Read the model definition and answer for the solid it produces. Units are mm, in the model's axes. Face numbers are marked on the shaded views. A direction names the side the tool comes from. Coordinates: 2 decimals unless noted, no trailing zeros. Write each loop counter-clockwise with the first axis right and the second up, starting at its lowest first coordinate (ties: lowest second). Pieces come first, ordered by that corner, then holes. Notation, with made-up numbers: (4, 3.25) - (14, 3.25) arc R16 cw to (14, 25.25) - close; hole circle Ø4 at (-2, 34). An arc over 180 degrees is marked (long way). Use a Markdown table: item, result.
from build123d import *

# Parameters (mm, degrees)
F1_DEPTH  = 230
F3_D      = 48.6
F5_D      = 6.5
F6_D      = 5.5
F7_SIZE   = 10
F9_D      = 13.72
F9_DEPTH  = 5
F11_D     = 19.05
F11_DEPTH = 5
F12_D     = 12.7
F12_DEPTH = 5


with BuildPart() as f1:
    # F0 (on Right) → F1 (new body)
    with BuildSketch(Plane.YZ):
        with BuildLine():
            Line((205, 0), (-205, 0))
            ThreePointArc((-205, 0), (-206.414214, -0.585786), (-207, -2))
            Line((-207, -2), (-207, -238))
            Line((-207, -238), (-247, -238))
            Line((-247, -238), (-247, -240))
            Line((-247, -240), (-207, -240))
            ThreePointArc((-207, -240), (-205.585786, -239.414214), (-205, -238))
            Line((-205, -238), (-205, -2))
            Line((-205, -2), (205, -2))
            Line((205, -2), (205, -238))
            ThreePointArc((205, -238), (205.585786, -239.414214), (207, -240))
            Line((207, -240), (247, -240))
            Line((247, -240), (247, -238))
            Line((247, -238), (207, -238))
            Line((207, -238), (207, -2))
            ThreePointArc((207, -2), (206.414214, -0.585786), (205, 0))
        make_face()
    extrude(amount=F1_DEPTH)

    # F3 (through all)
    with Locations(Plane.XY):
        with Locations((115, -162)):
            Hole(F3_D / 2)

    # F5 (through all)
    with Locations(Plane.XY.offset(-238)):
        with Locations((35, -237), (65, -237), (165, -237), (195, -237)):
            Hole(F5_D / 2)

    # F6 (through all)
    with Locations(Plane.XY.offset(-238)):
        with Locations((35, 237), (65, 237), (165, 237), (195, 237)):
            Hole(F6_D / 2)

    # F7
    f7_edges = [f1.edges().sort_by_distance(p)[0] for p in [
        (0, -247, -239),
        (230, -247, -239),
        (230, 247, -239),
        (0, 247, -239),
    ]]
    chamfer(f7_edges, length=F7_SIZE)

    # F9
    with Locations(Plane.XZ.offset(207)):
        with Locations((17.5, -20), (17.5, -200)):
            Hole(F9_D / 2, depth=F9_DEPTH)

    # F11
    with Locations(Plane(origin=(0, 207, 0), x_dir=(-1, 0, 0), z_dir=(0, 1, 0))):
        with Locations((-115, -20)):
            Hole(F11_D / 2, depth=F11_DEPTH)

    # F12
    with Locations(Plane(origin=(0, 207, 0), x_dir=(-1, 0, 0), z_dir=(0, 1, 0))):
        with Locations((-40, -20)):
            Hole(F12_D / 2, depth=F12_DEPTH)


solid = f1.part
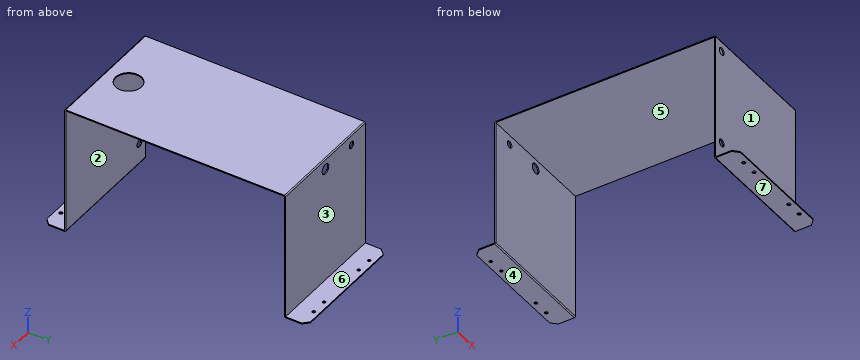
(1) A cutting plane is placed at D-D, the plane x = 182.5. Write down the section's boundary in (y, z), and give its area (3 significant figures).
Report:
| item | result |
|---|---|
| outline | (-247, -240) - (-207, -240) arc R2 ccw to (-205, -238) - (-205, -2) - (205, -2) - (205, -238) arc R2 ccw to (207, -240) - (247, -240) - (247, -238) - (207, -238) - (207, -2) arc R2 ccw to (205, 0) - (-205, 0) arc R2 ccw to (-207, -2) - (-207, -238) - (-247, -238) - close |
| area | 1,940 mm² |
(2) A cutting plane is placed at C-C, the plane z = -150. Write down the section's boundary in (x, y), and give its area (3 significant figures).
Report:
| item | result |
|---|---|
| outline | (0, -207) - (230, -207) - (230, -205) - (0, -205) - close; (0, 205) - (230, 205) - (230, 207) - (0, 207) - close |
| area | 920 mm² |
(3) A cutting plane is placed at A-A, the plane z = -20. Write down the section's boundary in (x, y) (3 decimals).
Report:
| item | result |
|---|---|
| outline | (0, -207) - (10.64, -207) - (10.64, -205) - (0, -205) - close; (0, 205) - (33.65, 205) - (33.65, 207) - (0, 207) - close; (24.36, -207) - (230, -207) - (230, -205) - (24.36, -205) - close; (46.35, 205) - (105.475, 205) - (105.475, 207) - (46.35, 207) - close; (124.525, 205) - (230, 205) - (230, 207) - (124.525, 207) - close |
(4) Straight lines are drawn through the part: L1, parallel to X at y = 237, z = -239.2; L2, parallel to Y at x = 79.5, z = -229; L3, parallel to X at y = -237, z = -238.9. For each, find the intervals that lie inside material, in ascending order.
Report:
| item | result |
|---|---|
| L1 | x = 0 to 32.25, 37.75 to 62.25, 67.75 to 162.25, 167.75 to 192.25, 197.75 to 230 |
| L2 | y = -207 to -205, 205 to 207 |
| L3 | x = 0 to 31.75, 38.25 to 61.75, 68.25 to 161.75, 168.25 to 191.75, 198.25 to 230 |
(5) The mould has two halves that part along Y. Classify the marked faces 1, 2, 3 and 4: pulls with the +Y half, pulls with the -Y half, needs draft (parallel to the pull), parting line crosses it, or undercut.
Report:
| item | result |
|---|---|
| face 1 | pulls with the -Y half |
| face 2 | undercut |
| face 3 | pulls with the +Y half |
| face 4 | needs draft |
(6) Each of these flat-tipped pins is pushed along its axis until it touches: P1, Ø5, axis at x = 165, y = 237, coming from the -Z side; P2, Ø10.5, axis at x = 165, y = -237, coming from the -Z side; P3, Ø10, axis at x = 155.5, z = -215, coming from the -Y side; P4, Ø6, axis at x = 160, z = -126, coming from the +Y side. Where does it stop, or does it pass through?
Report:
| item | result |
|---|---|
| P1 | passes through |
| P2 | stops at z = -240 |
| P3 | stops at y = -207 |
| P4 | stops at y = 207 |
(7) For the marked faces 5, 6 and 7, determine the directions among +Z, -Z, +X, -X, +Y, -Y from which every point of the face is accessible in a straight line to the end or side of a thin tool.
Report:
| item | result |
|---|---|
| face 5 | -Z, +X, -X |
| face 6 | +Z, +X, -X, +Y |
| face 7 | -Z, +X, -X, +Y, -Y |
(8) A cutting plane is placed at B-B, the plane x = 115. Write down the section's boundary in (y, z) (3 decimals).
Report:
| item | result |
|---|---|
| outline | (-247, -240) - (-207, -240) arc R2 ccw to (-205, -238) - (-205, -2) - (-186.3, -2) - (-186.3, 0) - (-205, 0) arc R2 ccw to (-207, -2) - (-207, -238) - (-247, -238) - close; (-137.7, -2) - (205, -2) - (205, -10.475) - (207, -10.475) - (207, -2) arc R2 ccw to (205, 0) - (-137.7, 0) - close; (205, -238) arc R2 ccw to (207, -240) - (247, -240) - (247, -238) - (207, -238) - (207, -29.525) - (205, -29.525) - close |
